```python
from build123d import *

# Parameters (mm, degrees)
BOSS_EXTRUDE1_DEPTH = 1.5
BOSS_EXTRUDE2_DEPTH = 5
SKETCH5_R           = 3
BOSS_EXTRUDE3_DEPTH = 5
SKETCH6_R           = 0.9
BOSS_EXTRUDE4_DEPTH = 3.3
FILLET1_R           = 0.5
SKETCH7_R           = 1.75
CUT_EXTRUDE1_DEPTH  = 2
SKETCH9_R           = 0.75
CUT_EXTRUDE2_DEPTH  = 5


with BuildPart() as part:
    # Sketch1 → Boss-Extrude1 (new body)
    with BuildSketch(Plane(origin=(0, 0, 0), x_dir=(1, 0, 0), z_dir=(0, 1, 0))):
        with BuildLine():
            Line((-22.5, -27.5), (22.5, -27.5))
            ThreePointArc((22.5, -27.5), (26.035533906, -26.035533906), (27.5, -22.5))
            Line((27.5, -22.5), (27.5, 22.5))
            ThreePointArc((27.5, 22.5), (26.035533906, 26.035533906), (22.5, 27.5))
            Line((22.5, 27.5), (-22.5, 27.5))
            ThreePointArc((-22.5, 27.5), (-26.035533906, 26.035533906), (-27.5, 22.5))
            Line((-27.5, 22.5), (-27.5, -22.5))
            ThreePointArc((-27.5, -22.5), (-26.035533906, -26.035533906), (-22.5, -27.5))
        make_face()
    extrude(amount=BOSS_EXTRUDE1_DEPTH)

    # Sketch2 → Boss-Extrude2 (add)
    with BuildSketch(Plane(origin=(0, 1.5, 0), x_dir=(1, 0, 0), z_dir=(0, 1, 0))):
        with BuildLine():
            Line((-27.5, 22.5), (-27.5, -22.5))
            ThreePointArc((-27.5, -22.5), (-26.035533906, -26.035533906), (-22.5, -27.5))
            Line((-22.5, -27.5), (22.5, -27.5))
            ThreePointArc((22.5, -27.5), (26.035533906, -26.035533906), (27.5, -22.5))
            Line((27.5, -22.5), (27.5, 22.5))
            ThreePointArc((27.5, 22.5), (26.035533906, 26.035533906), (22.5, 27.5))
            Line((22.5, 27.5), (-22.5, 27.5))
            ThreePointArc((-22.5, 27.5), (-26.035533906, 26.035533906), (-27.5, 22.5))
        make_face()
        with BuildLine():
            Line((-26, 22.5), (-26, -22.5))
            ThreePointArc((-26, -22.5), (-24.974873734, -24.974873734), (-22.5, -26))
            Line((-22.5, -26), (22.5, -26))
            ThreePointArc((22.5, -26), (24.974873734, -24.974873734), (26, -22.5))
            Line((26, -22.5), (26, 22.5))
            ThreePointArc((26, 22.5), (24.974873734, 24.974873734), (22.5, 26))
            Line((22.5, 26), (-22.5, 26))
            ThreePointArc((-22.5, 26), (-24.974873734, 24.974873734), (-26, 22.5))
        make_face(mode=Mode.SUBTRACT)
    extrude(amount=BOSS_EXTRUDE2_DEPTH)

    # Sketch5 → Boss-Extrude3 (add)
    with BuildSketch(Plane(origin=(0, 1.5, 0), x_dir=(1, 0, 0), z_dir=(0, 1, 0))):
        with Locations(Location((0, 0, 0), (0, 0, 90))):
            Circle(SKETCH5_R)
    extrude(amount=BOSS_EXTRUDE3_DEPTH)

    # Sketch6 → Boss-Extrude4 (add)
    # profile 1 of 4: a face of its own
    with BuildSketch(Plane(origin=(0, 1.5, 0), x_dir=(1, 0, 0), z_dir=(0, 1, 0))):
        with BuildLine():
            Line((-20.5, 26), (-20.5, 22.5))
            ThreePointArc((-20.5, 22.5), (-21.085786438, 21.085786438), (-22.5, 20.5))
            Line((-22.5, 20.5), (-26, 20.5))
            Line((-26, 20.5), (-26, 22.5))
            ThreePointArc((-26, 22.5), (-24.974873734, 24.974873734), (-22.5, 26))
            Line((-22.5, 26), (-20.5, 26))
        make_face()
        with Locations(Location((-22.5, 22.5, 0), (0, 0, 270))):
            Circle(SKETCH6_R, mode=Mode.SUBTRACT)
    # profile 2 of 4: a face of its own
    with BuildSketch(Plane(origin=(0, 1.5, 0), x_dir=(1, 0, 0), z_dir=(0, 1, 0))):
        with BuildLine():
            Line((22.5, 26), (20.5, 26))
            Line((20.5, 26), (20.5, 22.5))
            ThreePointArc((20.5, 22.5), (21.085786438, 21.085786438), (22.5, 20.5))
            Line((22.5, 20.5), (26, 20.5))
            Line((26, 20.5), (26, 22.5))
            ThreePointArc((26, 22.5), (24.974873734, 24.974873734), (22.5, 26))
        make_face()
        with Locations(Location((22.5, 22.5, 0), (0, 0, 90))):
            Circle(SKETCH6_R, mode=Mode.SUBTRACT)
    # profile 3 of 4: a face of its own
    with BuildSketch(Plane(origin=(0, 1.5, 0), x_dir=(1, 0, 0), z_dir=(0, 1, 0))):
        with BuildLine():
            Line((20.5, -26), (20.5, -22.5))
            ThreePointArc((20.5, -22.5), (21.085786438, -21.085786438), (22.5, -20.5))
            Line((22.5, -20.5), (26, -20.5))
            Line((26, -20.5), (26, -22.5))
            ThreePointArc((26, -22.5), (24.974873734, -24.974873734), (22.5, -26))
            Line((22.5, -26), (20.5, -26))
        make_face()
        with Locations(Location((22.5, -22.5, 0), (0, 0, 270))):
            Circle(SKETCH6_R, mode=Mode.SUBTRACT)
    # profile 4 of 4: a face of its own
    with BuildSketch(Plane(origin=(0, 1.5, 0), x_dir=(1, 0, 0), z_dir=(0, 1, 0))):
        with BuildLine():
            Line((-22.5, -26), (-20.5, -26))
            Line((-20.5, -26), (-20.5, -22.5))
            ThreePointArc((-20.5, -22.5), (-21.085786438, -21.085786438), (-22.5, -20.5))
            Line((-22.5, -20.5), (-26, -20.5))
            Line((-26, -20.5), (-26, -22.5))
            ThreePointArc((-26, -22.5), (-24.974873734, -24.974873734), (-22.5, -26))
        make_face()
        with Locations(Location((-22.5, -22.5, 0), (0, 0, 90))):
            Circle(SKETCH6_R, mode=Mode.SUBTRACT)
    extrude(amount=BOSS_EXTRUDE4_DEPTH)

    # Fillet1
    fillet1_edges = [part.edges().sort_by_distance(p)[0] for p in [
        (0, 6.5, 3),
    ]]
    fillet(fillet1_edges, radius=FILLET1_R)

    # Sketch7 → Cut-Extrude1 (cut)
    with BuildSketch(Plane.XZ):
        with Locations(Location((-22.5, 22.5, 0), (0, 0, 270))):
            Circle(SKETCH7_R)
        with Locations(Location((22.5, 22.5, 0), (0, 0, 90))):
            Circle(SKETCH7_R)
        with Locations(Location((22.5, -22.5, 0), (0, 0, 270))):
            Circle(SKETCH7_R)
        with Locations(Location((-22.5, -22.5, 0), (0, 0, 90))):
            Circle(SKETCH7_R)
    extrude(amount=-CUT_EXTRUDE1_DEPTH, mode=Mode.SUBTRACT)

    # Sketch9 → Cut-Extrude2 (cut, symmetric)
    with BuildSketch(Plane.XY):
        with Locations((-27.5, 5)):
            Circle(SKETCH9_R)
        with Locations((27.5, 5)):
            Circle(SKETCH9_R)
    extrude(amount=CUT_EXTRUDE2_DEPTH, both=True, mode=Mode.SUBTRACT)


solid = part.part
```
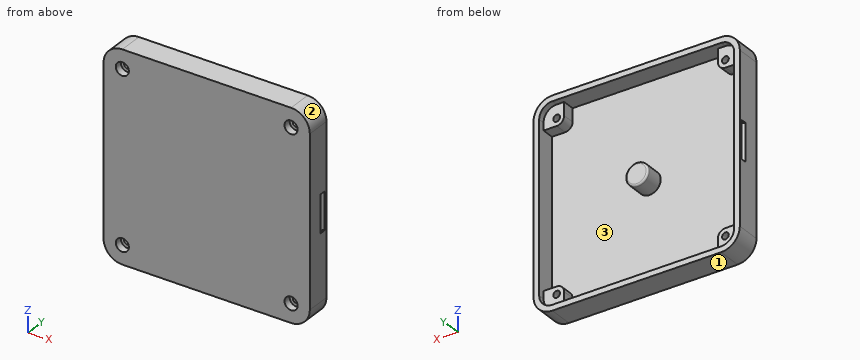
Here's how the part is built. I have some questions about the finished solid (model axes, mm). Face numbers are marked on the shaded views. Coordinates: 2 decimals unless noted, no trailing zeros. Write each loop counter-clockwise with the first axis right and the second up, starting at its lowest first coordinate (ties: lowest second). Pieces come first, ordered by that corner, then holes. Notation, with made-up numbers: (45, 74) - (73, 74) arc R24 ccw to (73, 88) - close; hole circle Ø1 at (-4, 79.5). An arc over 180 degrees is marked (long way). One line per item, written item: value.
1) I'm going to push flat-ended pins straight in: P1, Ø3, axis at x = -22.5, z = 22.5, coming from the -Y side; P2, Ø2.5, axis at x = -22.5, z = -22.5, coming from the +Y side; P3, Ø5, axis at x = 12.5, z = 13, coming from the +Y side. Where does each tip first touch, or does it pass through?
Model answer:
P1: stops at y = 2
P2: stops at y = 4.8
P3: stops at y = 1.5
2) We'd pull the mould along Z, two halves only. Please class the marked faces 1, 2 and 3: pulls with the +Z half, pulls with the -Z half, needs draft (parallel to the pull), parting line crosses it, or undercut.
Model answer:
face 1: pulls with the -Z half
face 2: pulls with the +Z half
face 3: undercut
3) Suppose I cut it at A-A on y = 3. State how many separate pieces and enclosed holes the cut face has, and give its area (3 significant figures).
Model answer:
separate pieces: 2
enclosed holes: 5
area: 435 mm²
4) I need wall thicknesses on line 1 along X through (y, z) = (2.85, -22.5); line 2 along X through (y, z) = (1.1, -22.5). Which ranges of each line are inside material? Lowest first, please.
Model answer:
line 1: x = -27.5 to -23.4, -21.6 to -20.5, 20.5 to 21.6, 23.4 to 27.5
line 2: x = -27.5 to -24.25, -20.75 to 20.75, 24.25 to 27.5
5) Suppose I cut it at D-D on z = 15.5. Write out the boundary of the cut face in (x, y), and give its area (3 significant figures).
Model answer:
outline: (-27.5, 0) - (27.5, 0) - (27.5, 6.5) - (26, 6.5) - (26, 1.5) - (-26, 1.5) - (-26, 6.5) - (-27.5, 6.5) - close
area: 97.5 mm²
6) Suppose I cut it at C-C on x = 0. Write out the boundary of the cut face in (y, z).
Model answer:
outline: (0, -27.5) - (6.5, -27.5) - (6.5, -26) - (1.5, -26) - (1.5, -3) - (6, -3) arc R0.5 ccw to (6.5, -2.5) - (6.5, 2.5) arc R0.5 ccw to (6, 3) - (1.5, 3) - (1.5, 26) - (6.5, 26) - (6.5, 27.5) - (0, 27.5) - close
7) Suppose I cut it at B-B on z = 0. Write out the boundary of the cut face in (x, y), and give its area (3 significant figures).
Model answer:
outline: (-27.5, 0) - (27.5, 0) - (27.5, 4.25) arc R0.75 cw to (27.5, 5.75) - (27.5, 6.5) - (26, 6.5) - (26, 1.5) - (3, 1.5) - (3, 6) arc R0.5 ccw to (2.5, 6.5) - (-2.5, 6.5) arc R0.5 ccw to (-3, 6) - (-3, 1.5) - (-26, 1.5) - (-26, 6.5) - (-27.5, 6.5) - (-27.5, 5.75) arc R0.75 cw to (-27.5, 4.25) - close
area: 126 mm²
